CAD build for the part. Positions are in the model's coordinates, mm. Face numbers are marked on the shaded views. Give positions to 0.01 mm unless a question says otherwise; leave off trailing zeros. Loops run counter-clockwise (first coordinate to the right, second up) from the corner with the lowest first, then second, coordinate; pieces in that order, holes last.
```python
from build123d import *

# Parameters (mm, degrees)
F1_DEPTH = 483.87
F2_R     = 63.5
F3_DEPTH = 137.16
F4_R     = 127
F5_R     = 38.1
F6_DEPTH = 81.28
F7_R     = 127


with BuildPart() as f1:
    # F0 (on Front) → F1 (new body)
    with BuildSketch(Plane.XZ):
        with BuildLine():
            Line((-396.698482, -189.28613), (873.301518, -189.28613))
            Line((873.301518, -189.28613), (873.301518, -141.02613))
            Line((873.301518, -141.02613), (-418.627456, -141.02613))
            ThreePointArc((-418.627456, -141.02613), (-456.18836, -108.736454), (-461.409152, -59.480104))
            Line((-461.409152, -59.480104), (-12.396346, 389.532702))
            Line((-12.396346, 389.532702), (-46.521319, 423.657675))
            Line((-46.521319, 423.657675), (-495.534125, -25.355131))
            ThreePointArc((-495.534125, -25.355131), (-492.408796, -135.230838), (-396.698482, -189.28613))
        make_face()
    extrude(amount=F1_DEPTH)

    # F2 (on face) → F3 (cut)
    with BuildSketch(Plane.XY.offset(-141.02613)):
        with BuildLine():
            Line((441.501518, -305.435), (695.501518, -305.435))
            ThreePointArc((695.501518, -305.435), (759.001518, -241.935), (695.501518, -178.435))
            Line((695.501518, -178.435), (441.501518, -178.435))
            ThreePointArc((441.501518, -178.435), (378.001518, -241.935), (441.501518, -305.435))
        make_face()
        with Locations((60.501518, -241.935)):
            Circle(F2_R)
    extrude(amount=-F3_DEPTH, mode=Mode.SUBTRACT)

    # F4
    f4_edges = [f1.edges().sort_by_distance(p)[0] for p in [
        (873.301518, -483.87, -165.15613),
        (873.301518, 0, -165.15613),
    ]]
    fillet(f4_edges, radius=F4_R)

    # F5 (on face) → F6 (cut)
    with BuildSketch(Plane(origin=(-235.089497, 0, 235.089497), x_dir=(0, -1, 0), z_dir=(-0.707107, 0, 0.707107))):
        with Locations((369.57, 76.175675)):
            Circle(F5_R)
        with Locations((114.3, 76.175675)):
            Circle(F5_R)
    extrude(amount=-F6_DEPTH, mode=Mode.SUBTRACT)

    # F7
    f7_edges = [f1.edges().sort_by_distance(p)[0] for p in [
        (-29.458833, -483.87, 406.595189),
        (-29.458833, 0, 406.595189),
    ]]
    fillet(f7_edges, radius=F7_R)


solid = f1.part
```
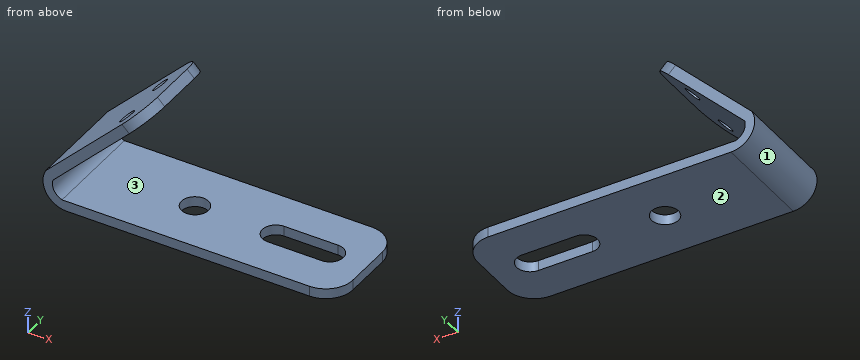
1. Saw through at A-A, the plane x = 637. List the corners of the cut face in (y, z) (3 decimals).
Responses:
outline: (-483.87, -189.286) - (-305.435, -189.286) - (-305.435, -141.026) - (-483.87, -141.026) - close; (-178.435, -189.286) - (0, -189.286) - (0, -141.026) - (-178.435, -141.026) - close
2. Saw through at C-C, the plane y = -383. List the corners of the cut face in (x, z).
Responses:
outline: (-495.53, -25.36) arc R111.76 ccw to (-396.7, -189.29) - (870.58, -189.29) - (870.58, -141.03) - (-418.63, -141.03) arc R67.18 cw to (-461.41, -59.48) - (-172.31, 229.62) - (-206.44, 263.74) - close; (-156.01, 314.17) - (-121.89, 280.04) - (-14.32, 387.61) - (-48.44, 421.74) - close
3. Saw through at D-D, the plane x = -275.5. List the corners of the cut face in (y, z), and give its area (3 significant figures).
Responses:
outline: (-483.87, -189.29) - (0, -189.29) - (0, -141.03) - (-483.87, -141.03) - close; (-483.87, 126.43) - (0, 126.43) - (0, 194.68) - (-483.87, 194.68) - close
area: 56,400 mm2
4. Pull direction Z, two halves, no side cores. Call the marked faces 1, 2 and 3: released by +Z, released by -Z, zero draft, split by the parting line, or undercut.
Responses:
face 1: split by the parting line
face 2: released by -Z
face 3: undercut
5. Saw through at B-B, the plane y = -203. List the corners of the cut face in (x, z).
Responses:
outline: (-495.53, -25.36) arc R111.76 ccw to (-396.7, -189.29) - (10.34, -189.29) - (10.34, -141.03) - (-418.63, -141.03) arc R67.18 cw to (-461.41, -59.48) - (-12.4, 389.53) - (-46.52, 423.66) - close; (110.66, -189.29) - (391.34, -189.29) - (391.34, -141.03) - (110.66, -141.03) - close; (745.66, -189.29) - (873.3, -189.29) - (873.3, -141.03) - (745.66, -141.03) - close
6. Probe line 1 along Z through (x, y) = (365.5, -325); line 2 along Z through (x, y) = (-146.5, -247.5); line 3 along Z through (x, y) = (-364, -330.5). List the from-to ranges inside material, lowest first.
Responses:
line 1: z = -189.29 to -141.03
line 2: z = -189.29 to -141.03, 255.43 to 323.68
line 3: z = -189.29 to -141.03, 37.93 to 106.18
7. Drop flat-ended pins along their axis: pin 1 (4 mm diameter, centred on y = -389.5, z = 76.5, fed in from +X); pin 2 (2 mm diameter, centred on x = -71, y = -396, fed in from +Z). Give the stop position or say it passes through.
Responses:
pin 1: stops at x = -323.43
pin 2: stops at z = 400.18
